CAD build for the part. Positions are in the model's coordinates, mm. A direction names the side the tool comes from. Round coordinates to 2 decimals unless told otherwise and drop trailing zeros. Write each loop counter-clockwise with the first axis right and the second up, starting at its lowest first coordinate (ties: lowest second). Pieces come first, ordered by that corner, then holes. Notation, with made-up numbers: (13.25, -29) - (19.25, -29) arc R20 ccw to (19.25, -21) - close; hole circle Ø9 at (10.25, -26). An arc over 180 degrees is marked (long way). Put each result on its own line as item: value. Start each with the question number.
Item 1: Cut at A-A (z = 24). Give the cut face in (x, y), and give its area (3 significant figures).
Item 2: Cut at D-D (x = 19). Give the cut face in (y, z).
Item 3: 3-axis set-ups, long thin cutter, end or side, ignore diameter. For faces 1 (the flat face through (-115, -15, -1)), 2 (the flat face through (11, -30, 1)), 3 (the cylindrical face through (-182.975, 2.348, -52.148)), 4 (the flat face through (75, 34, -30)), 5 (the flat face through (75, 34, 10)): which of +Z, -Z, +X, -X, +Y, -Y reach the whole face in a straight line?
Item 4: Cut at B-B (y = -15). Give the cut face in (x, z).
Item 5: Drill centre lines: line 1 (Y direction, x = 75, z = -26); line 2 (X direction, y = 50, z = -13.75); line 3 (Y direction, x = -188, z = -40). Where is each one in solid material? Low to high. Write a range as from..to.
Item 6: Pin check, flat tips, straight feed: pin 1 Ø22.5 at (x, y) = (75, 50) entering from +Z; pin 2 Ø10 at (x, y) = (90, 19.5) entering from -Z; pin 3 Ø16 at (y, z) = (40, 16.5) entering from -X; pin 4 Ø25 at (x, y) = (66, 38) entering from +Z. Stop position of each tip, or through.
Item 7: Mould opens along X. For faces 6 (the flat face through (-1, 25, -1)), 7 (the cylindrical face through (74.45, 74.994, 20.14)), 8 (the flat face through (-86, 4, -55)) say: released by +X, released by -X, zero draft, split by the parting line, or undercut.
Item 8: Cut at C-C (x = 75). Give the cut face in (y, z), and give its area (3 significant figures).
```python
from build123d import *

# Parameters (mm, degrees)
BOSS_EXTRUDE1_DEPTH = 30
BOSS_EXTRUDE2_DEPTH = 30
SKETCH2_5_W         = 200
SKETCH2_5_H         = 30
BOSS_EXTRUDE3_DEPTH = 75
SKETCH2_6_W         = 200
SKETCH2_6_H         = 30
BOSS_EXTRUDE4_DEPTH = 75
SKETCH3_R           = 12.5
BOSS_EXTRUDE5_DEPTH = 20
BOSS_EXTRUDE6_START = -20
SKETCH4_R           = 12.5
BOSS_EXTRUDE6_DEPTH = 20
BOSS_EXTRUDE7_DEPTH = 25
BOSS_EXTRUDE8_DEPTH = 25
SKETCH7_W           = 150
SKETCH7_H           = 30
BOSS_EXTRUDE9_DEPTH = 25
FILLET1_R           = 10


with BuildPart() as part:
    # Sketch2 → Boss-Extrude1 (new body)
    with BuildSketch(Plane.XY):
        Polygon((100, 25), (-100, 25), (-122.855339059, 47.855339059), (-165.355339059, 5.355339059), (-215.355339059, 5.355339059), (-215.355339059, -30), (-130, -30), (-100, 0), (100, 0), align=None)
    extrude(amount=BOSS_EXTRUDE1_DEPTH)

    # Sketch2_4 → Boss-Extrude2 (add)
    with BuildSketch(Plane.XY):
        Polygon((100, 25), (-100, 25), (-122.855339059, 47.855339059), (-165.355339059, 5.355339059), (-215.355339059, 5.355339059), (-215.355339059, -30), (-130, -30), (-100, 0), (100, 0), align=None)
    extrude(amount=-BOSS_EXTRUDE2_DEPTH)

    # Sketch2_5 → Boss-Extrude3 (add)
    with BuildSketch(Plane.XY):
        with Locations((0, -15)):
            Rectangle(SKETCH2_5_W, SKETCH2_5_H)
    extrude(amount=BOSS_EXTRUDE3_DEPTH)

    # Sketch2_6 → Boss-Extrude4 (add)
    with BuildSketch(Plane.XY):
        with Locations((0, -15)):
            Rectangle(SKETCH2_6_W, SKETCH2_6_H)
    extrude(amount=-BOSS_EXTRUDE4_DEPTH)

    # Sketch3 → Boss-Extrude5 (add)
    with BuildSketch(Plane.XY.offset(30)):
        with BuildLine():
            Line((100, 25), (50, 25))
            Line((50, 25), (50, 50))
            ThreePointArc((50, 50), (75, 75), (100, 50))
            Line((100, 50), (100, 25))
        make_face()
        with Locations((75, 50)):
            Circle(SKETCH3_R, mode=Mode.SUBTRACT)
    extrude(amount=-BOSS_EXTRUDE5_DEPTH)

    # Sketch4 → Boss-Extrude6 (add)
    with BuildSketch(Plane(origin=(0, 0, -30), x_dir=(-1, 0, 0), z_dir=(0, 0, -1)).offset(BOSS_EXTRUDE6_START)):
        with BuildLine():
            Line((-100, 25), (-50, 25))
            Line((-50, 25), (-50, 50))
            ThreePointArc((-50, 50), (-75, 75), (-100, 50))
            Line((-100, 50), (-100, 25))
        make_face()
        with Locations(Location((-75, 50, 0), (0, 0, 180))):
            Circle(SKETCH4_R, mode=Mode.SUBTRACT)
    extrude(amount=BOSS_EXTRUDE6_DEPTH)

    # Sketch5 → Boss-Extrude7 (add)
    with BuildSketch(Plane(origin=(0, 0, -30), x_dir=(-1, 0, 0), z_dir=(0, 0, -1))):
        Polygon((122.855339059, 47.855339059), (100, 25), (-100, 25), (-100, 0), (100, 0), (130, -30), (215.355339059, -30), (215.355339059, 5.355339059), (165.355339059, 5.355339059), align=None)
    extrude(amount=BOSS_EXTRUDE7_DEPTH)

    # Sketch6 → Boss-Extrude8 (add)
    with BuildSketch(Plane.XY.offset(30)):
        Polygon((-122.855339059, 47.855339059), (-100, 25), (100, 25), (100, 0), (-100, 0), (-130, -30), (-215.355339059, -30), (-215.355339059, 5.355339059), (-165.355339059, 5.355339059), align=None)
    extrude(amount=BOSS_EXTRUDE8_DEPTH)

    # Sketch7 → Boss-Extrude9 (add)
    with BuildSketch(Plane(origin=(100, 0, 0), x_dir=(0, 0, -1), z_dir=(1, 0, 0))):
        with Locations((0, -15)):
            Rectangle(SKETCH7_W, SKETCH7_H)
    extrude(amount=BOSS_EXTRUDE9_DEPTH)

    # Fillet1
    fillet1_edges = [part.edges().sort_by_distance(p)[0] for p in [
        (-144.105339059, 26.605339059, -55),
        (-111.42766953, 36.42766953, -55),
        (0, 25, -55),
        (-215.355339059, -12.32233047, -55),
        (-190.355339059, 5.355339059, -55),
        (-144.105339059, 26.605339059, 55),
        (-190.355339059, 5.355339059, 55),
        (-215.355339059, -12.32233047, 55),
        (0, 25, 55),
        (-111.42766953, 36.42766953, 55),
        (125, -15, 75),
        (125, -15, -75),
        (125, 0, 0),
        (-215.355339059, 5.355339059, 0),
        (-122.855339059, 47.855339059, 0),
        (12.5, 0, 75),
        (-100, -15, 75),
        (12.5, 0, -75),
        (-100, -15, -75),
    ]]
    fillet(fillet1_edges, radius=FILLET1_R)


solid = part.part
```
Output values:
1. outline: (-215.36, -30) - (-130, -30) - (-100, 0) - (-100, -30) - (125, -30) - (125, -10) arc R10 ccw to (115, 0) - (100, 0) - (100, 50) arc R25 ccw to (50, 50) - (50, 25) - (-100, 25) - (-115.78, 40.78) arc R10 ccw to (-129.93, 40.78) - (-165.36, 5.36) - (-205.36, 5.36) arc R10 ccw to (-215.36, -4.64) - close; hole circle Ø25 at (75, 50)
1. area: 18,700 mm2
2. outline: (-30, -75) - (-10, -75) arc R10 ccw to (0, -65) - (0, -55) - (15, -55) arc R10 ccw to (25, -45) - (25, 45) arc R10 ccw to (15, 55) - (0, 55) - (0, 65) arc R10 ccw to (-10, 75) - (-30, 75) - close
3. face 1: +Z, -Z, -Y
3. face 2: +Z, -Z, +X, -X, -Y
3. face 3: -Z, -X, +Y
3. face 4: -Z, +X, +Y
3. face 5: +X, +Y
4. outline: (-215.36, -45) arc R10 ccw to (-205.36, -55) - (-115, -55) - (-115, 55) - (-205.36, 55) arc R10 ccw to (-215.36, 45) - close; (-100, -65) arc R10 ccw to (-90, -75) - (115, -75) arc R10 ccw to (125, -65) - (125, 65) arc R10 ccw to (115, 75) - (-90, 75) arc R10 ccw to (-100, 65) - close
5. line 1: -30..37.5, 62.5..75
5. line 2: 50..62.5, 87.5..100
5. line 3: -30..5.36
6. pin 1: through
6. pin 2: z = -55
6. pin 3: x = -138.71
6. pin 4: z = 30
7. face 6: undercut
7. face 7: split by the parting line
7. face 8: zero draft
8. outline: (-30, -75) - (-10, -75) arc R10 ccw to (0, -65) - (0, -55) - (15, -55) arc R10 ccw to (25, -45) - (25, -30) - (37.5, -30) - (37.5, -10) - (25, -10) - (25, 10) - (37.5, 10) - (37.5, 30) - (25, 30) - (25, 45) arc R10 ccw to (15, 55) - (0, 55) - (0, 65) arc R10 ccw to (-10, 75) - (-30, 75) - close; (62.5, -30) - (75, -30) - (75, -10) - (62.5, -10) - close; (62.5, 10) - (75, 10) - (75, 30) - (62.5, 30) - close
8. area: 8,160 mm2
